from build123d import *

# Parameters (mm, degrees)
EXTRUDE_1_DEPTH = 10
SKETCH_3_W      = 10
SKETCH_3_H      = 14.4
EXTRUDE_2_DEPTH = 17
FILLET_1_R      = 20


with BuildPart() as part:
    # 草图1 → 凸台-拉伸1 (new body)
    with BuildSketch(Plane.XY):
        Polygon((0, 0), (-35, 0), (0, 14.4), align=None)
    extrude(amount=EXTRUDE_1_DEPTH)

    # 草图3 → 凸台-拉伸2 (add)
    with BuildSketch(Plane(origin=(0, 0, 0), x_dir=(0, 0, -1), z_dir=(1, 0, 0))):
        with Locations((-5, 7.2)):
            Rectangle(SKETCH_3_W, SKETCH_3_H)
    extrude(amount=EXTRUDE_2_DEPTH)

    # 圆角1
    fillet_1_edges = [part.edges().sort_by_distance(p)[0] for p in [
        (0, 14.4, 5),
    ]]
    fillet(fillet_1_edges, radius=FILLET_1_R)


solid = part.part
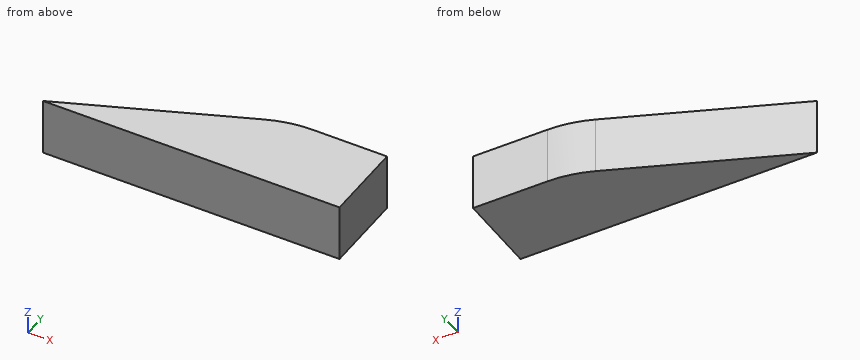
Part model, mm, in its own coordinate system. Coordinates: 2 decimals unless noted, no trailing zeros. Write each loop counter-clockwise with the first axis right and the second up, starting at its lowest first coordinate (ties: lowest second). Pieces come first, ordered by that corner, then holes. Notation, with made-up numbers: M 55.5,19.25 L 111.5,19.25 A18 ccw 111.5,30.25 Z; hole C 23,84.25 d6. An arc over 180 degrees is marked long. Return JSON: item names as keys, results as strings.
1. Flat gauge pins, fed straight in: pin 1 Ø1 at (x, z) = (-7, 7.5) entering from +Y; pin 2 Ø4 at (y, z) = (5.5, 5) entering from -X; pin 3 Ø6 at (y, z) = (4.5, 8) entering from -X. Where does each tip first touch, or does it go through?
Determined:
{"pin 1": "y = 11.73", "pin 2": "x = -26.49", "pin 3": "x = -31.35"}
2. Saw through at B-B, the plane x = -21. Write the cut outline in (y, z), then the cut area to 3 significant figures.
Determined:
{"outline": "M 0,0 L 5.76,0 L 5.76,10 L 0,10 Z", "area": "57.6 mm²"}
3. Probe L1, parallel to X at y = 6.75, z = 7.25; L2, parallel to X at y = 1, z = 8.75; L3, parallel to Y at x = -0.5, z = 2.5. List the from-to ranges inside material, lowest first.
Determined:
{"L1": "-18.59 to 17", "L2": "-32.57 to 17", "L3": "0 to 13.9"}
4. Saw through at A-A, the plane z = 6.5. Write the cut outline in (x, y), then the cut area to 3 significant figures.
Determined:
{"outline": "M -35,0 L 17,0 L 17,14.4 L 3.95,14.4 A20 ccw -3.66,12.9 Z", "area": "496 mm²"}
5. Saw through at C-C, the plane y = 6. Write the cut outline in (x, z), then the cut area to 3 significant figures.
Determined:
{"outline": "M -20.42,0 L 17,0 L 17,10 L -20.42,10 Z", "area": "374 mm²"}
